```python
from build123d import *

# Parameters (mm, degrees)
SKETCH1_W                 = 10
SKETCH1_H                 = 10
BOSS_EXTRUDE1_DEPTH       = 5
M3X0_5_TAPPED_HOLE1_D     = 2.5
M3X0_5_TAPPED_HOLE1_DEPTH = 6.748924226
M3X0_5_TAPPED_HOLE1_TIP   = 0.751075774


with BuildPart() as part:
    # Sketch1 → Boss-Extrude1 (new body, symmetric)
    with BuildSketch(Plane.XY):
        Rectangle(SKETCH1_W, SKETCH1_H)
    extrude(amount=BOSS_EXTRUDE1_DEPTH, both=True)

    # M3x0.5 Tapped Hole1
    with Locations(Plane(origin=(0, -5, 0), x_dir=(-1, 0, 0), z_dir=(0, -1, 0))):
        with Locations((-2.5, 0), (2.5, 0)):
            Hole(M3X0_5_TAPPED_HOLE1_D / 2, depth=M3X0_5_TAPPED_HOLE1_DEPTH)
            with Locations((0, 0, -(M3X0_5_TAPPED_HOLE1_DEPTH + M3X0_5_TAPPED_HOLE1_TIP / 2))):  # 118° drill point
                Cone(0, M3X0_5_TAPPED_HOLE1_D / 2, M3X0_5_TAPPED_HOLE1_TIP, mode=Mode.SUBTRACT)


solid = part.part
```
Model file for the job. Use its own axes, mm. A direction names the side the tool comes from. Coordinates: 2 decimals unless noted, no trailing zeros. Order: outer loops, then holes, each group sorted by start corner. A loop starts at its lowest first (then second) coordinate and runs counter-clockwise, first axis right, second up. Notation, with made-up numbers: (87.25, 33) -> (110.25, 33) arc R23 cw to (110.25, 60) -> close; hole circle Ø1 at (27.5, 58). An arc over 180 degrees is marked (long way). Answer as a JSON object with one key per item and string values. Group by question number.
1) Flat gauge pin, fed straight in: pin 1 (6 mm diameter, centred on x = -3, z = 0.5, fed in from -Y). Where does the tip first touch, or does it go through?
2) Pull direction X, two halves, no side cores. Call faces 3 (the face through (-2.28, 2.37, -0.01)), 4 (the face through (-5, 0, 0)), 5 (the face through (0, 0, -5)): +X half, -X half, draft (parallel to the pull), parting line (faces both ways), or undercut.
3) Which spindle directions (+Z, -Z, +X, -X, +Y, -Y) get a long thin tool onto all of the face, cutting with end or side? Do faces 1 (the face through (3.69, -1.58, -0.38)), 2 (the face through (0, 0, 5)). Say none if no direction does.
4) Cut at A-A, the plane y = -3. Write the cut outline in (x, z), then the cut area to 3 significant figures.
5) Drill centre lines: L1, parallel to X at y = -0.25, z = -0.75; L2, parallel to Z at x = 2.5, y = -0.5; L3, parallel to Z at x = -1.5, y = -0.25. Where is each one in solid material? Low to high.
Check values:
{
 "1": {"pin 1": "stops at y = -5"},
 "2": {"face 3": "undercut", "face 4": "-X half", "face 5": "draft"},
 "3": {"face 1": "-Y", "face 2": "+Z, +X, -X, +Y, -Y"},
 "4": {"outline": "(-5, -5) -> (5, -5) -> (5, 5) -> (-5, 5) -> close; hole circle Ø2.5 at (-2.5, 0); hole circle Ø2.5 at (2.5, 0)", "area": "90.2 mm²"},
 "5": {"L1": "x = -5 to -3.5, -1.5 to 1.5, 3.5 to 5", "L2": "z = -5 to -1.25, 1.25 to 5", "L3": "z = -5 to -0.75, 0.75 to 5"}
}
